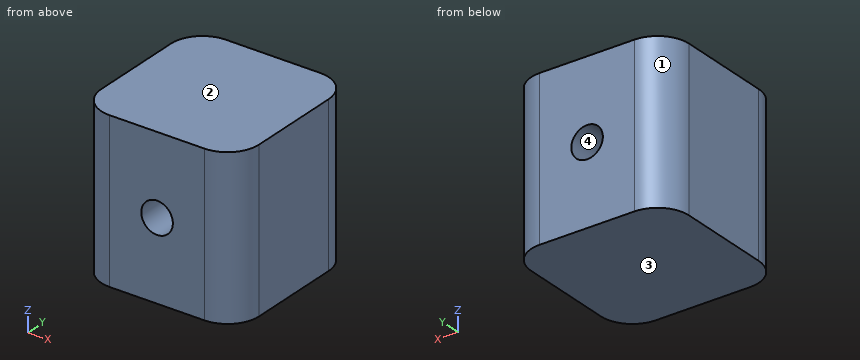
```python
from build123d import *

# Parameters (mm, degrees)
F1_DEPTH = 127
F2_R     = 25.4
F3_R     = 12.7
F4_DEPTH = 127.001


with BuildPart() as f1:
    # F0 (on Top) → F1 (new body)
    with BuildSketch(Plane.XY):
        with BuildLine():
            Line((70.322224, 68.553888), (-31.277776, 68.553888))
            ThreePointArc((-31.277776, 68.553888), (-49.238288, 61.1144), (-56.677776, 43.153888))
            Line((-56.677776, 43.153888), (-56.677776, -58.446112))
            Line((-56.677776, -58.446112), (70.322224, -58.446112))
            Line((70.322224, -58.446112), (70.322224, 68.553888))
        make_face()
    extrude(amount=F1_DEPTH)

    # F2
    f2_edges = [f1.edges().sort_by_distance(p)[0] for p in [
        (70.322224, 68.553888, 63.5),
        (70.322224, -58.446112, 63.5),
        (-56.677776, -58.446112, 63.5),
    ]]
    fillet(f2_edges, radius=F2_R)

    # F3 (on face) → F4 (cut, through all)
    with BuildSketch(Plane.XZ.offset(58.446112)):
        with Locations((6.822224, 63.5)):
            Circle(F3_R)
    extrude(amount=-F4_DEPTH, mode=Mode.SUBTRACT)


solid = f1.part
```
Could you check a few things on this model? Use its own coordinates, in mm. Face numbers are marked on the shaded views. Give positions to 0.01 mm unless a question says otherwise; leave off trailing zeros. Order: outer loops, then holes, each group sorted by start corner. A loop starts at its lowest first (then second) coordinate and runs counter-clockwise, first axis right, second up.
Q1. Suppose I cut it at B-B, the plane x = 16.5. Write out the boundary of the cut face in (y, z), and give its area (3 significant figures).
Q2. I'm going to push a flat-ended pin straight in: P1, Ø12, axis at y = 51, z = 65.5, coming from the -X side. Where does the tip first touch, or does it pass through?
Q3. Suppose I cut it at D-D, the plane z = 116. Write out the boundary of the cut face in (x, y).
Q4. We'd pull the mould along Z, two halves only. Please class the marked faces 1, 2, 3 and 4: +Z half, -Z half, draft (parallel to the pull), parting line (faces both ways), or undercut.
Q5. Suppose I cut it at C-C, the plane y = 12. Write out the boundary of the cut face in (x, z), and give its area (3 significant figures).
Q6. If I drill on line 1 along X through (y, z) = (-30, 63); line 2 along Z through (x, y) = (0.5, 63); line 3 along Z through (x, y) = (0, 52), over which ranges is the centre line in solid material (lowest first)?
Q7. Suppose I cut it at A-A, the plane z = 63.5. Write out the boundary of the cut face in (x, y).
Solution:
1. outline: (-58.45, 0) - (68.55, 0) - (68.55, 55.28) - (-58.45, 55.28) - close; (-58.45, 71.72) - (68.55, 71.72) - (68.55, 127) - (-58.45, 127) - close
1. area: 14,000 mm2
2. P1: stops at x = -56.61
3. outline: (-56.68, -33.05) arc R25.4 ccw to (-31.28, -58.45) - (44.92, -58.45) arc R25.4 ccw to (70.32, -33.05) - (70.32, 43.15) arc R25.4 ccw to (44.92, 68.55) - (-31.28, 68.55) arc R25.4 ccw to (-56.68, 43.15) - close
4. face 1: draft
4. face 2: +Z half
4. face 3: -Z half
4. face 4: undercut
5. outline: (-56.68, 0) - (70.32, 0) - (70.32, 127) - (-56.68, 127) - close; hole circle Ø25.4 at (6.82, 63.5)
5. area: 15,600 mm2
6. line 1: x = -56.68 to -5.87, 19.51 to 70.32
6. line 2: z = 0 to 52.49, 74.51 to 127
6. line 3: z = 0 to 52.79, 74.21 to 127
7. outline: (-56.68, -33.05) arc R25.4 ccw to (-31.28, -58.45) - (-5.88, -58.45) - (-5.88, 68.55) - (-31.28, 68.55) arc R25.4 ccw to (-56.68, 43.15) - close; (19.52, -58.45) - (44.92, -58.45) arc R25.4 ccw to (70.32, -33.05) - (70.32, 43.15) arc R25.4 ccw to (44.92, 68.55) - (19.52, 68.55) - close
